from build123d import *

# Parameters (mm, degrees)
F0_W     = 50.8
F0_H     = 25.4
F1_DEPTH = 3.175
F2_R     = 8.25
F3_DEPTH = 25.4
F4_W     = 10.16
F4_H     = 5.08
F4_W_2   = 10.142652
F4_H_2   = 1.381879
F5_DEPTH = 25.4
F6_R     = 1.27


with BuildPart() as f1:
    # F0 (on Top) → F1 (new body)
    with BuildSketch(Plane.XY):
        Rectangle(F0_W, F0_H)
    extrude(amount=F1_DEPTH)

    # F2 (on face) → F3 (cut)
    with BuildSketch(Plane.XY.offset(3.175)):
        with Locations((-12.7, 0)):
            Circle(F2_R)
        with Locations((12.7, 0)):
            Circle(F2_R)
    extrude(amount=-F3_DEPTH, mode=Mode.SUBTRACT)

    # F4 (on face) → F5 (cut)
    with BuildSketch(Plane.XY.offset(3.175)):
        with Locations((0, 10.16)):
            Rectangle(F4_W, F4_H)
        with Locations((-0.022494, -12.009061)):
            Rectangle(F4_W_2, F4_H_2)
    extrude(amount=-F5_DEPTH, mode=Mode.SUBTRACT)

    # F6
    f6_edges = [f1.edges().sort_by_distance(p)[0] for p in [
        (-5.08, 7.62, 1.5875),
        (5.08, 7.62, 1.5875),
    ]]
    fillet(f6_edges, radius=F6_R)


solid = f1.part
Model file for the job. Use its own axes, mm. A direction names the side the tool comes from. Give positions to 0.01 mm unless a question says otherwise; leave off trailing zeros. Write each loop counter-clockwise with the first axis right and the second up, starting at its lowest first coordinate (ties: lowest second). Pieces come first, ordered by that corner, then holes. Notation, with made-up numbers: M 3.5,42.25 L 59.5,42.25 A22 cw 59.5,50.25 Z; hole C -22,53 d5. An arc over 180 degrees is marked long. One line per item, written item: value. Start each with the question number.
Q1. Two-plate mould, pull along Y, no slides. Class faces 1 (the cylindrical face through (4.458, 0.363, 1.61)), 2 (the flat face through (25.4, 0, 2)), 3 (the flat face through (0, -11.318, 2)): +Y half, -Y half, draft (parallel to the pull), parting line (faces both ways), or undercut.
Q2. Saw through at B-B, the plane y = 0. Write the cut outline in (x, z) (3 decimals).
Q3. Saw through at C-C, the plane x = 12.7. Write the cut outline in (y, z) (3 decimals).
Q4. 3-axis set-ups, long thin cutter, end or side, ignore diameter. For faces 4 (the flat face through (15, 12.7, 2)), 5 (the cylindrical face through (-4.718, 8.002, 1.565)), 6 (the flat face through (-5.094, -12, 2)): which of +Z, -Z, +X, -X, +Y, -Y reach the whole face in a straight line?
Q5. Probe probe 1 along X at (y, z) = (1.5, 0.45); probe 2 along X at (y, z) = (7.25, 2.95); probe 3 along Y at (x, z) = (12.7, 2.3). List the from-to ranges inside material, lowest first. Write a range as [from, to].
Q6. Saw through at A-A, the plane z = 2.7. Write the cut outline in (x, y).
Q7. Drop flat-ended pins along their axis: pin 1 Ø1 at (x, z) = (1, 1) entering from -Y; pin 2 Ø1.6 at (x, z) = (0, 2) entering from +Y; pin 3 Ø15 at (x, y) = (-12.7, 0) entering from +Z. Give the stop position or say it passes through.
Q8. Saw through at D-D, the plane x = -17.5. Write the cut outline in (y, z) (3 decimals).
Output values:
1. face 1: undercut
1. face 2: draft
1. face 3: -Y half
2. outline: M -25.4,0 L -20.95,0 L -20.95,3.175 L -25.4,3.175 Z; M -4.45,0 L 4.45,0 L 4.45,3.175 L -4.45,3.175 Z; M 20.95,0 L 25.4,0 L 25.4,3.175 L 20.95,3.175 Z
3. outline: M -12.7,0 L -8.25,0 L -8.25,3.175 L -12.7,3.175 Z; M 8.25,0 L 12.7,0 L 12.7,3.175 L 8.25,3.175 Z
4. face 4: +Z, -Z, +X, -X, +Y
4. face 5: +Z, -Z, +Y
4. face 6: +Z, -Z, -Y
5. probe 1: x = [-25.4, -20.81], [-4.59, 4.59], [20.81, 25.4]
5. probe 2: x = [-25.4, -16.64], [-8.76, 8.76], [16.64, 25.4]
5. probe 3: y = [-12.7, -8.25], [8.25, 12.7]
6. outline: M -25.4,-12.7 L -5.09,-12.7 L -5.09,-11.32 L 5.05,-11.32 L 5.05,-12.7 L 25.4,-12.7 L 25.4,12.7 L 5.08,12.7 L 5.08,8.89 A1.27 cw 3.81,7.62 L -3.81,7.62 A1.27 cw -5.08,8.89 L -5.08,12.7 L -25.4,12.7 Z; hole C -12.7,0 d16.5; hole C 12.7,0 d16.5
7. pin 1: stops at y = -11.32
7. pin 2: stops at y = 7.62
7. pin 3: passes through
8. outline: M -12.7,0 L -6.71,0 L -6.71,3.175 L -12.7,3.175 Z; M 6.71,0 L 12.7,0 L 12.7,3.175 L 6.71,3.175 Z
